Autodesk Inventor part; units mm, degrees
ref_plane "YZ Plane" through (0, 0, 0) normal (1, 0, 0) x (0, 1, 0)
ref_plane "XZ Plane" through (0, 0, 0) normal (0, 1, 0) x (-1, 0, 0)
ref_plane "XY Plane" through (0, 0, 0) normal (0, 0, 1) x (1, 0, 0)
sketch "Sketch1" plane through (0, 0, 0) normal (1, 0, 0) x (0, 1, 0)
  line L0 (6.35, 12.7) -> (-65.1002, 12.7)
  line L1 (-65.1002, 12.7) -> (-65.1002, -147.6502)
  line L2 (-65.1002, -147.6502) -> (6.35, -147.6502)
  line L3 (6.35, -147.6502) -> (6.35, 12.7)
  point P0 (0, 0)
  dimension "d0" = 71.4502
  dimension "d1" = 160.3502
extrude "Extrusion1" add sketch "Sketch1" along normal blind 6.35
sketch "Sketch2" plane through (6.35, 0, 0) normal (1, 0, 0) x (0, 0, -1)
  circle A0 centre (66.675, -28.575) radius 7.9375
  point P0 (0, 0)
  dimension "d4" = 15.875
extrude "Extrusion2" add sketch "Sketch2" along normal blind 10.16
properties part number "lid3" material "PMMA Plastic"
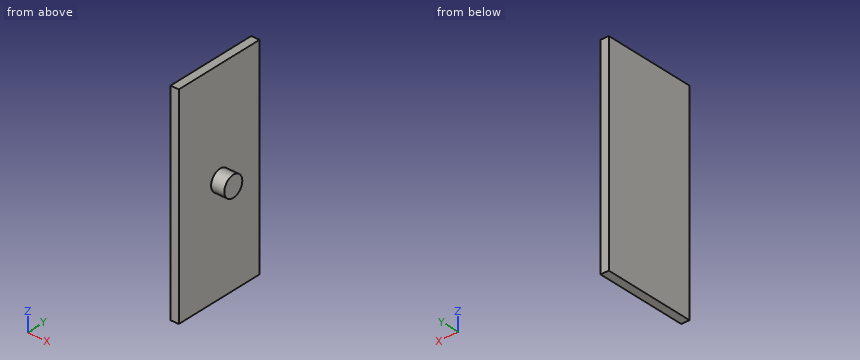
Verification items for the finished model (mm, model axes). Give positions to 0.01 mm unless a question says otherwise; leave off trailing zeros. Order: outer loops, then holes, each group sorted by start corner. A loop starts at its lowest first (then second) coordinate and runs counter-clockwise, first axis right, second up. Notation, with made-up numbers: (68, -27.5) - (117, -27.5) arc R8 ccw to (117, -23.5) - close; hole circle Ø1 at (57.5, 74.25). An arc over 180 degrees is marked (long way). Answer as CSV lines item,"result". Start each with the question number.
Item 1: Section check A-A, the plane y = -31. Record the boundary of the cut face in (x, z), plus the area to 3 significant figures.
Item 2: Section check C-C, the plane z = -128.5. Record the boundary of the cut face in (x, y).
Item 3: Gauge pin test, flat ends, axial feed: pin 1 (12 mm diameter, centred on y = -35, z = -118, fed in from -X); pin 2 (6 mm diameter, centred on y = -37, z = -14, fed in from +X). Record the tip position at first contact, or that the pin passes through.
Item 4: Material ranges on L1, parallel to X at y = -32.5, z = -18, recorded low to high.
Item 5: Section check D-D, the plane y = -23. Record the boundary of the cut face in (x, z).
Item 6: Section check B-B, the plane x = 12. Record the boundary of the cut face in (y, z) (1 decimal), plus the area to 3 significant figures.
Filled in:
1,outline,"(0, -147.65) - (6.35, -147.65) - (6.35, -74.23) - (16.51, -74.23) - (16.51, -59.12) - (6.35, -59.12) - (6.35, 12.7) - (0, 12.7) - close"
1,area,"1,170 mm^2"
2,outline,"(0, -65.1) - (6.35, -65.1) - (6.35, 6.35) - (0, 6.35) - close"
3,pin 1,"x = 0"
3,pin 2,"x = 6.35"
4,L1,"0 to 6.35"
5,outline,"(0, -147.65) - (6.35, -147.65) - (6.35, -72.33) - (16.51, -72.33) - (16.51, -61.02) - (6.35, -61.02) - (6.35, 12.7) - (0, 12.7) - close"
6,outline,"circle Ø15.9 at (-28.6, -66.7)"
6,area,"198 mm^2"
